from build123d import *

# Parameters (mm, degrees)
F0_W      = 106
F0_H      = 166
F1_DEPTH  = 295
F2_T      = -3
F3_R      = 2
F4_DEPTH  = 150
F5_R      = 2
F6_DEPTH  = 125
F7_R      = 4
F8_DEPTH  = 52
F9_R      = 4
F10_DEPTH = 82


with BuildPart() as f1:
    # F0 (on Top) → F1 (new body)
    with BuildSketch(Plane.XY):
        Rectangle(F0_W, F0_H)
    extrude(amount=F1_DEPTH)

    # F2
    f2_openings = [f1.faces().sort_by_distance(p)[0] for p in [
        (0, 0, 295),
    ]]
    offset(amount=F2_T, openings=f2_openings)

    # F3 (on Right) → F4 (cut)
    with BuildSketch(Plane.YZ):
        with Locations((-16, 287)):
            Circle(F3_R)
        with Locations((16, 287)):
            Circle(F3_R)
        with Locations((-75, 8)):
            Circle(F3_R)
    extrude(amount=F4_DEPTH, mode=Mode.SUBTRACT)

    # F5 (on Front) → F6 (cut, symmetric)
    with BuildSketch(Plane.XZ):
        with Locations((-5, 287)):
            Circle(F5_R)
    extrude(amount=F6_DEPTH, both=True, mode=Mode.SUBTRACT)

    # F7 (on Right) → F8 (cut)
    with BuildSketch(Plane.YZ):
        with Locations((-16, 287)):
            Circle(F7_R)
        with Locations((16, 287)):
            Circle(F7_R)
    extrude(amount=F8_DEPTH, mode=Mode.SUBTRACT)

    # F9 (on Front) → F10 (cut, symmetric)
    with BuildSketch(Plane.XZ):
        with Locations((-5, 287)):
            Circle(F9_R)
    extrude(amount=F10_DEPTH, both=True, mode=Mode.SUBTRACT)


solid = f1.part
Verification items for the finished model (mm, model axes). A direction names the side the tool comes from. Give positions to 0.01 mm unless a question says otherwise; leave off trailing zeros. Order: outer loops, then holes, each group sorted by start corner. A loop starts at its lowest first (then second) coordinate and runs counter-clockwise, first axis right, second up. Notation, with made-up numbers: M 57,-2 L 78,-2 A6 cw 78,2 Z; hole C 4,-10 d8. An arc over 180 degrees is marked long. Use one line per item in the form item = value. Start each with the question number.
Q1. Go/stop test with flat-tipped pins: pin 1 Ø12 at (x, y) = (5.5, -65) entering from +Z; pin 2 Ø8 at (x, y) = (-0.5, -19) entering from -Z; pin 3 Ø3 at (y, z) = (16, 287) entering from +X. Record where each tip stops, or that it passes through.
Q2. Section check B-B (x = -30.5). Enter the section's corners in (y, z).
Q3. Section check C-C (y = -55). Enter the section's corners in (x, z).
Q4. Scan lines: line 1 along Y through (x, z) = (50.5, 287); line 2 along Y through (x, z) = (-3, 160.5); line 3 along Y through (x, z) = (52.6, 287). Record each from-to range of solid material in increasing order. Write a range as [from, to].
Q5. Access from +Z, -Z, +X, -X, +Y, -Y to the whole of each face (thin tool, end or side, straight path). Record for faces 5 (the cylindrical face through (-3.154, 80.986, 283.451)), 6 (the flat face through (-53, -1, 145)), 7 (the flat face through (-50, -1, 147)).
Q6. Section check A-A (z = 144.5). Enter the section's corners in (x, y), then the cut area to 3 significant figures.
Q7. Mould release check, pull along Y, two halves, no side actions. Record for faces 1 (the cylindrical face through (50.986, 17.846, 283.451)), 2 (the flat face through (-1, 1, 0)), 3 (the flat face through (-1, 83, 145)), 4 (the flat face through (-7, 82, 286)): +Y half, -Y half, draft (parallel to the pull), parting line (faces both ways), or undercut.
Evaluation:
q1.pin_1 = 3
q1.pin_2 = 0
q1.pin_3 = -50
q2.outline = M -83,0 L 83,0 L 83,295 L 80,295 L 80,3 L -80,3 L -80,295 L -83,295 Z
q3.outline = M -53,0 L 53,0 L 53,295 L 50,295 L 50,3 L -50,3 L -50,295 L -53,295 Z
q4.line_1 = [-83, -20], [-12, 12], [20, 83]
q4.line_2 = [-83, -80], [80, 83]
q4.line_3 = [-83, -18], [-14, 14], [18, 83]
q5.face_5 = none
q5.face_6 = +Z, -Z, -X, +Y, -Y
q5.face_7 = +Z
q6.outline = M -53,-83 L 53,-83 L 53,83 L -53,83 Z; hole M -50,-80 L 50,-80 L 50,80 L -50,80 Z
q6.area = 1,600 mm2
q7.face_1 = undercut
q7.face_2 = draft
q7.face_3 = +Y half
q7.face_4 = undercut
